Input: part model. Units: mm. Frame: model coordinates. Face numbers are marked on the shaded views. A direction names the side the tool comes from. Coordinates: 2 decimals unless noted, no trailing zeros. Write each loop counter-clockwise with the first axis right and the second up, starting at its lowest first coordinate (ties: lowest second). Pieces come first, ordered by that corner, then holes.
1) Section query A-A (x = 0). Output: boundary loops of the cut face in (y, z), then the cut area to 3 significant figures.
2) Section query C-C (z = 4.5). Output: boundary loops of the cut face in (x, y).
3) Set-up query: the marked faces 5 and 6. Return all of +Z, -Z, +X, -X, +Y, -Y with unobstructed straight access to the full face (end or side cutting, diameter ignored); none if empty.
4) Pin query (flat end, axial travel): pin 1 Ø4 at (x, z) = (-3.5, 4) entering from -Y; pin 2 Ø3 at (x, z) = (8, 5.5) entering from -Y; pin 3 Ø6.5 at (x, y) = (0, 0) entering from -Z; pin 4 Ø1.5 at (y, z) = (-7, 5) entering from +X. Return the tip coordinate at first contact, or that it passes through.
5) Draft query along X for the marked faces 1, 2, 3 and 4. Return one class per face: pulls with the +X half, pulls with the -X half, needs draft (parallel to the pull), parting line crosses it, or undercut.
6) Line query: L1, parallel to Y at x = 0, z = 0.1; L2, parallel to Y at x = 5, z = 6.75; L3, parallel to Y at x = 0.5, z = 1.5. Output: solid intervals per line, ascending.
Autodesk Inventor part; units mm, degrees
ref_plane "Work Plane1" through (0, 0, 3.5) normal (0, 0, 1) x (1, 0, 0)
ref_plane "YZ Plane" through (0, 0, 0) normal (1, 0, 0) x (0, 1, 0)
ref_plane "XZ Plane" through (0, 0, 0) normal (0, 1, 0) x (-1, 0, 0)
sketch "Sketch1" plane through (0, 0, 0) normal (0, 0, 1) x (1, 0, 0)
  circle A0 centre (0, 0) radius 4
  circle A1 centre (0, 0) radius 11
  dimension "d0" = 8
  dimension "d1" = 22
extrude "Extrusion1" add sketch "Sketch1" along normal blind 7
sketch "Sketch2" plane through (0, 0, 7) normal (0, 0, 1) x (1, 0, 0)
  circle A0 centre (0, 0) radius 11
  circle A1 centre (0, 0) radius 4
  circle A2 centre (0, 0) radius 9.5
  circle A3 centre (0, 0) radius 5.5
  dimension "d4" = 1.5
  dimension "d5" = 1.5
extrude "Extrusion2" cut sketch "Sketch2" against normal blind 0.5 contours A2
ref_plane "Work Plane1" through (0, 0, 3.5) normal (0, 0, 1) x (1, 0, 0)
mirror "Mirror1" about plane through (0, 0, 3.5) normal (0, 0, 1) of "Extrusion2"
chamfer "Chamfer1" distance 0.2 angle 45 2 edges at (-11, 0, 7) (-11, 0, 0)
properties part number "608 Bearing"
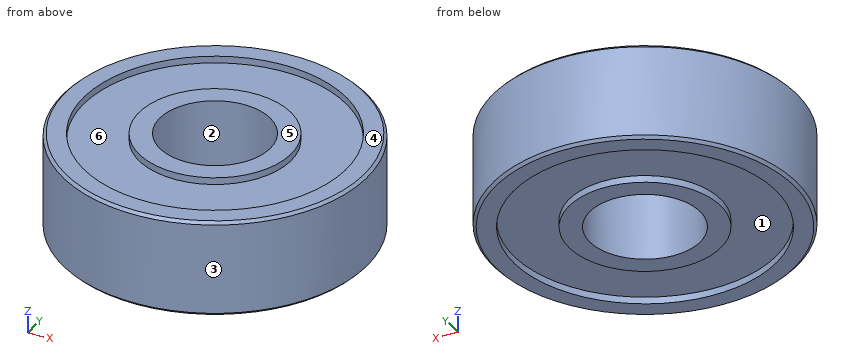
Answer:
1. outline: (-11, 0.2) - (-10.8, 0) - (-9.5, 0) - (-9.5, 0.5) - (-5.5, 0.5) - (-5.5, 0) - (-4, 0) - (-4, 7) - (-5.5, 7) - (-5.5, 6.5) - (-9.5, 6.5) - (-9.5, 7) - (-10.8, 7) - (-11, 6.8) - close; (4, 0) - (5.5, 0) - (5.5, 0.5) - (9.5, 0.5) - (9.5, 0) - (10.8, 0) - (11, 0.2) - (11, 6.8) - (10.8, 7) - (9.5, 7) - (9.5, 6.5) - (5.5, 6.5) - (5.5, 7) - (4, 7) - close
1. area: 89.9 mm2
2. outline: circle Ø22 at (0, 0); hole circle Ø8 at (0, 0)
3. face 5: +Z, +X, -X, +Y, -Y
3. face 6: +Z
4. pin 1: stops at y = -10.9
4. pin 2: stops at y = -8.87
4. pin 3: passes through
4. pin 4: stops at x = 9.05
5. face 1: undercut
5. face 2: undercut
5. face 3: parting line crosses it
5. face 4: needs draft
6. L1: y = -10.9 to -9.5, -5.5 to -4, 4 to 5.5, 9.5 to 10.9
6. L2: y = -9.8 to -8.08, -2.29 to 2.29, 8.08 to 9.8
6. L3: y = -10.99 to -3.97, 3.97 to 10.99
